```python
from build123d import *

# Parameters (mm, degrees)
SKETCH_1_R           = 110
SKETCH_1_R_2         = 1.15
EXTRUDE_1_DEPTH      = 1
SKETCH_2_R           = 6
SKETCH_2_R_2         = 1.15
EXTRUDE_2_DEPTH      = 5
EXTRUDE_2_DEPTH_BACK = 6
SKETCH_3_R           = 1
CUT_EXTRUDE_1_DEPTH  = 25


with BuildPart() as part:
    # 草图1 → 凸台-拉伸1 (new body)
    with BuildSketch(Plane.XY):
        Circle(SKETCH_1_R)
        Circle(SKETCH_1_R_2, mode=Mode.SUBTRACT)
    extrude(amount=EXTRUDE_1_DEPTH)

    # 草图2 → 凸台-拉伸2 (add, two sides)
    with BuildSketch(Plane(origin=(0, 0, 0), x_dir=(-1, 0, 0), z_dir=(0, 0, -1))) as extrude_2_sk:
        Circle(SKETCH_2_R)
        Circle(SKETCH_2_R_2, mode=Mode.SUBTRACT)
    extrude(amount=EXTRUDE_2_DEPTH)
    extrude(extrude_2_sk.sketch, amount=-EXTRUDE_2_DEPTH_BACK)

    # 草图3 → 切除-拉伸1 (cut, symmetric)
    with BuildSketch(Plane(origin=(0, 0, 0), x_dir=(1, 0, 0), z_dir=(0, 1, 0))):
        with Locations((0, 2.5)):
            Circle(SKETCH_3_R)
        with Locations((0, -3.5)):
            Circle(SKETCH_3_R)
    extrude(amount=CUT_EXTRUDE_1_DEPTH, both=True, mode=Mode.SUBTRACT)


solid = part.part
```
Could you check a few things on this model? Use its own coordinates, in mm. A direction names the side the tool comes from. Round coordinates to 2 decimals unless told otherwise and drop trailing zeros. Loops run counter-clockwise (first coordinate to the right, second up) from the corner with the lowest first, then second, coordinate; pieces in that order, holes last. Notation, with made-up numbers: M -27.5,30.25 L 7.5,30.25 A33 ccw 7.5,60.25 Z; hole C 23.5,75.5 d8. An arc over 180 degrees is marked long. Answer as CSV lines item,"result".
1) Imagine slicing it at B-B on y = 39. List the corners of the cut face in (x, z) for me, and give its area (3 significant figures).
From the geometry:
outline,"M -102.85,0 L 102.85,0 L 102.85,1 L -102.85,1 Z"
area,"206 mm^2"
2) Which directions (+Z, -Z, +X, -X, +Y, -Y) give clear straight access to the entire face, cutting with the end or side of a thin tool? Please do faces 1 (the flat face through (0.1, 1.4, 6)), 2 (the cylindrical face through (1.301, -5.857, -2.465)), 3 (the cylindrical face through (1.301, -5.857, 3.465)).
From the geometry:
face 1,"+Z, +X, -X, +Y, -Y"
face 2,"-Z"
face 3,"+Z"
3) Imagine slicing it at A-A on x = 86.5. List the corners of the cut face in (y, z) for me, and give its area (3 significant figures).
From the geometry:
outline,"M -67.95,0 L 67.95,0 L 67.95,1 L -67.95,1 Z"
area,"136 mm^2"
4) If I drill on probe 1 along Z at (x, y) = (0, 4.4); probe 2 along Z at (x, y) = (37, 76.5); probe 3 along X at (y, z) = (-1.8, -2.5), over which ranges is the centre line in solid material (lowest first)?
From the geometry:
probe 1,"-5 to -3.5, -1.5 to 2.5, 4.5 to 6"
probe 2,"0 to 1"
probe 3,"-5.72 to -1, 1 to 5.72"
5) For pin 1 Ø3 at (x, y) = (-78, -15) entering from -Z; pin 2 Ø1.5 at (y, z) = (-0.5, -3.5) entering from +X; pin 3 Ø2.5 at (x, z) = (0, 3.5) entering from +Y, each with a flat end and sliding along its axis, tell me the tip position at first contact or that it passes through.
From the geometry:
pin 1,"z = 0"
pin 2,"x = 6"
pin 3,"y = 6"
